Study the drawing (mm; zero at the part's minimum x, y, z) and answer. A direction names the side the tool comes from. Round coordinates to 2 decimals unless told otherwise and drop trailing zeros. Order: outer loops, then holes, each group sorted by start corner. A loop starts at its lowest first (then second) coordinate and runs counter-clockwise, first axis right, second up. Notation, with made-up numbers: (57, -37.75) - (68, -37.75) arc R28 ccw to (68, -19.75) - close; hole circle Ø5 at (55.25, 15.25). An arc over 180 degrees is marked (long way). Put each result on its own line as item: value.
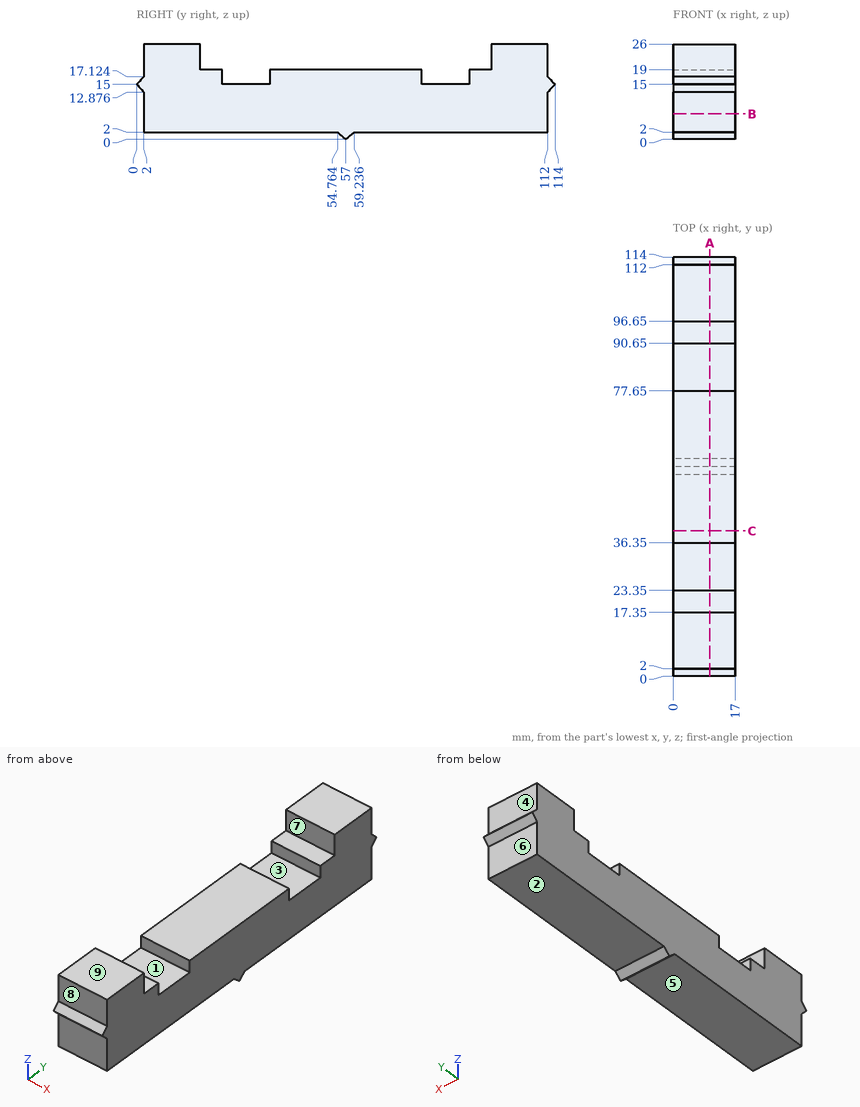
1) Given pin 1 Ø6 at (y, z) = (93.5, 4) entering from -X; pin 2 Ø1.5 at (x, z) = (4.5, 9) entering from +Y; pin 3 Ø6.5 at (x, y) = (6, 92.5) entering from +Z; pin 4 Ø5 at (x, y) = (4.5, 22) entering from -Z, each flat-ended and moving along its own axis, determine where each tip first touches the part or whether it passes through.
Findings below:
pin 1: stops at x = 0
pin 2: stops at y = 112
pin 3: stops at z = 19
pin 4: stops at z = 2
2) A cutting plane is placed at C-C on y = 39.5. Write down the section's boundary in (x, z), then the cut area to 3 significant figures.
Findings below:
outline: (0, 2) - (17, 2) - (17, 19) - (0, 19) - close
area: 289 mm2
3) For a pull along Y with two mould halves and no side action, classify the marked faces 1, 2, 3 and 4 as pulls with the +Y half, pulls with the -Y half, needs draft (parallel to the pull), parting line crosses it, or undercut.
Findings below:
face 1: undercut
face 2: needs draft
face 3: undercut
face 4: pulls with the +Y half
4) A cutting plane is placed at A-A on x = 10. Write down the section's boundary in (y, z).
Findings below:
outline: (0, 15) - (2, 12.88) - (2, 2) - (54.76, 2) - (57, 0) - (59.24, 2) - (112, 2) - (112, 12.88) - (114, 15) - (112, 17.12) - (112, 26) - (96.65, 26) - (96.65, 19) - (90.65, 19) - (90.65, 15) - (77.65, 15) - (77.65, 19) - (36.35, 19) - (36.35, 15) - (23.35, 15) - (23.35, 19) - (17.35, 19) - (17.35, 26) - (2, 26) - (2, 17.12) - close
5) Straight lines are drawn through the part: L1, parallel to Y at x = 11, z = 18.25; L2, parallel to Y at x = 8, z = 22; L3, parallel to Y at x = 13, z = 7. For each, find the intervals that lie inside material, in ascending order. Write a range as from..to.
Findings below:
L1: y = 2..23.35, 36.35..77.65, 90.65..112
L2: y = 2..17.35, 96.65..112
L3: y = 2..112
6) A cutting plane is placed at B-B on z = 7. Write down the section's boundary in (x, y), then the cut area to 3 significant figures.
Findings below:
outline: (0, 2) - (17, 2) - (17, 112) - (0, 112) - close
area: 1,870 mm2
7) For the marked faces 5, 6, 7, 8 and 9, determine the directions among +Z, -Z, +X, -X, +Y, -Y from which every point of the face is accessible in a straight line to the end or side of a thin tool.
Findings below:
face 5: -Z, +X, -X, -Y
face 6: -Z, +X, -X, +Y
face 7: +Z, +X, -X
face 8: +Z, +X, -X, -Y
face 9: +Z, +X, -X, +Y, -Y
